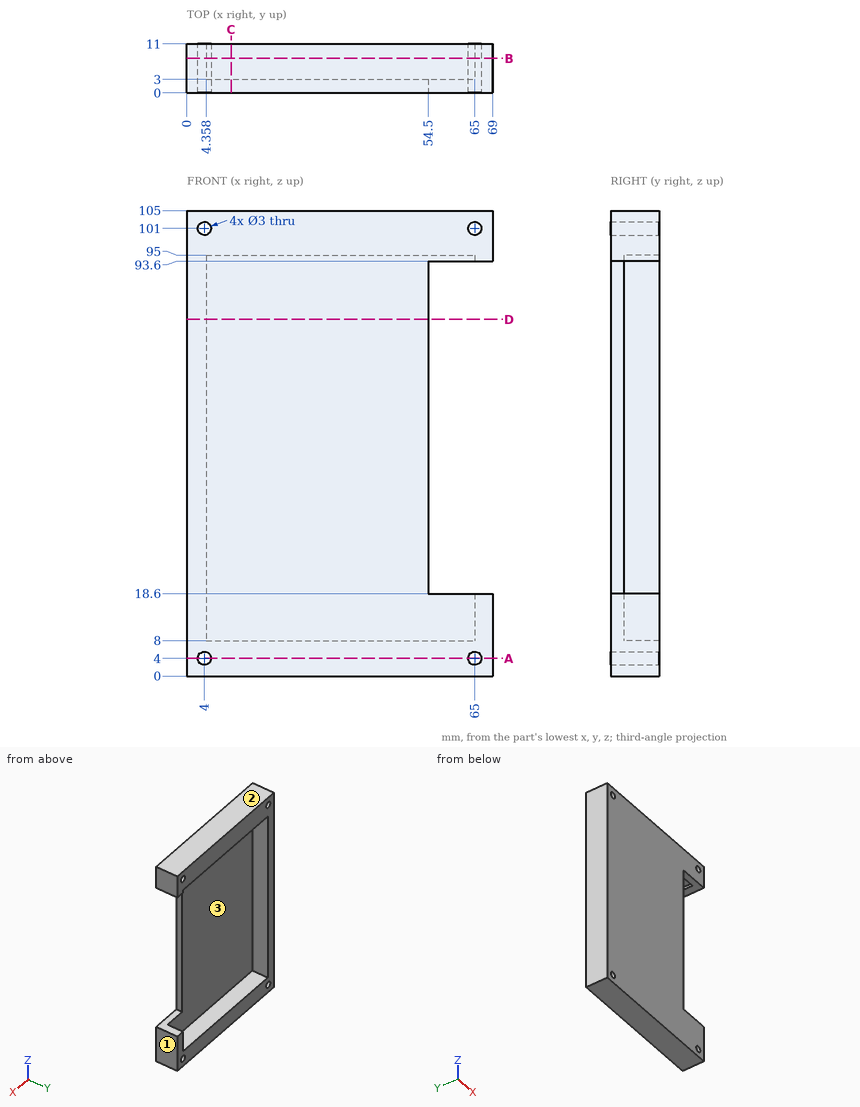
Source: three-view drawing plus pictorial views. Frame: mm from the lowest corner of the part. Round coordinates to 2 decimals unless told otherwise and drop trailing zeros. Loops run counter-clockwise (first coordinate to the right, second up) from the corner with the lowest first, then second, coordinate; pieces in that order, holes last.
Q1. Section A-A, the plane z = 4. Return loops of the section in (x, y).
Q2. Mould query, pull axis X, two halves, no side actions, for the marked faces 1, 2 and 3. Classes: pulls with the +X half, pulls with the -X half, needs draft (parallel to the pull), parting line crosses it, or undercut.
Q3. Section C-C, the plane x = 10. Return loops of the section in (y, z).
Q4. Section D-D, the plane z = 80.5. Return loops of the section in (x, y).
Q5. Ray query, line 1 (X direction, y = 7.5, z = 101); line 2 (Z direction, x = 38, y = 7.25); line 3 (Z direction, x = 4, y = 4.5). Return the intervals inside material, ascending.
Q6. First-contact query: P1, Ø5, axis at x = 46.5, z = 15.5, coming from the +Y side; P2, Ø1.8, axis at x = 4, z = 101, coming from the -Y side; P3, Ø1.5, axis at y = 1, z = 44, coming from the +X side; P4, Ø2.5, axis at y = 9, z = 45.5, coming from the +X side. Flat tips, straight axial feed; report the tip coordinate or a pass-through.
Q7. Section B-B, the plane y = 7.75. Return loops of the section in (x, z), plus the area to 3 significant figures.
Solutions:
1. outline: (0, 0) - (2.5, 0) - (2.5, 11) - (0, 11) - close; (5.5, 0) - (63.5, 0) - (63.5, 11) - (5.5, 11) - close; (66.5, 0) - (69, 0) - (69, 11) - (66.5, 11) - close
2. face 1: pulls with the +X half
2. face 2: needs draft
2. face 3: undercut
3. outline: (0, 0) - (11, 0) - (11, 8) - (3, 8) - (3, 95) - (11, 95) - (11, 105) - (0, 105) - close
4. outline: (0, 0) - (54.5, 0) - (54.5, 3) - (4.36, 3) - (4.36, 11) - (0, 11) - close
5. line 1: x = 0 to 2.5, 5.5 to 63.5, 66.5 to 69
5. line 2: z = 0 to 8, 95 to 105
5. line 3: z = 0 to 2.5, 5.5 to 99.5, 102.5 to 105
6. P1: stops at y = 3
6. P2: passes through
6. P3: stops at x = 54.5
6. P4: stops at x = 4.36
7. outline: (0, 0) - (69, 0) - (69, 18.6) - (65, 18.6) - (65, 8) - (4.36, 8) - (4.36, 95) - (65, 95) - (65, 93.6) - (69, 93.6) - (69, 105) - (0, 105) - close; hole circle Ø3 at (4, 4); hole circle Ø3 at (4, 101); hole circle Ø3 at (65, 4); hole circle Ø3 at (65, 101)
7. area: 1,640 mm2
